Input: part model. Units: mm. Frame: model coordinates. A direction names the side the tool comes from. Coordinates: 2 decimals unless noted, no trailing zeros. Write each loop counter-clockwise with the first axis right and the second up, starting at its lowest first coordinate (ties: lowest second). Pieces come first, ordered by that corner, then holes. Notation, with made-up numbers: (51, -3.75) -> (106, -3.75) arc R19 cw to (106, 12.25) -> close; hole circle Ø11 at (28, 42.5). An arc over 180 degrees is marked (long way). Use one line per item in the form item = value. Start each with the question number.
(1) Set-up query: faces 1 (the face through (71.451, 4.504, -16.574)), 2 (the face through (-71.451, 4.504, 16.574)), 3 (the face through (1, 5, 7.5)), 4 (the face through (-1, 10, -11)). Return all of +Z, -Z, +X, -X, +Y, -Y with unobstructed straight access to the full face (end or side cutting, diameter ignored); none if empty.
(2) Cut plane A-A on z = 0. Return the cut outline in (x, y).
(3) Cut plane B-B on x = 31. Return the cut outline in (y, z), plus the area to 3 significant figures.
(4) First-contact query: pin 1 (3 mm diameter, centred on y = 5, z = 15, fed in from +X); pin 2 (3 mm diameter, centred on y = 5, z = 15, fed in from -X). Flat tips, straight axial feed; report the tip coordinate or a pass-through.
(5) Ray query, line 1 along Z through (x, y) = (71.5, 5); line 2 along Y through (x, z) = (-72.75, -15); line 3 along Z through (x, y) = (-36, 5). Return the intervals inside material, ascending.
(6) Pull-direction query (Z, two-part tool) for faces 5 (the face through (-75, 5, 0)), 6 (the face through (-67.2, 5.1, -15.3)), 7 (the face through (-1, 5, -7.5)), 8 (the face through (-1, 5, -25)); classes: released by +Z, released by -Z, zero draft, split by the parting line, or undercut.
```python
from build123d import *

# Parameters (mm, degrees)
SKETCH_1_W                       = 150
SKETCH_1_H                       = 50
EXTRUDE_1_DEPTH                  = 10
CUT_EXTRUDE_1_DEPTH              = 10
HOLE_WIZARD_M4_1_D               = 3.3
HOLE_WIZARD_M4_1_DEPTH           = 7
HOLE_WIZARD_M4_1_TIP             = 0.991420021
HOLE_WIZARD_M4_2_D               = 3.3
HOLE_WIZARD_M4_2_DEPTH           = 7
HOLE_WIZARD_M4_2_TIP             = 0.991420021
HOLE_WIZARD_M4_2_ON_FACE_2_D     = 3.3
HOLE_WIZARD_M4_2_ON_FACE_2_DEPTH = 7
HOLE_WIZARD_M4_2_ON_FACE_2_TIP   = 0.991420021


with BuildPart() as part:
    # 草图1 → 凸台-拉伸1 (new body)
    with BuildSketch(Plane(origin=(0, 0, 0), x_dir=(1, 0, 0), z_dir=(0, 1, 0))):
        Rectangle(SKETCH_1_W, SKETCH_1_H)
    extrude(amount=EXTRUDE_1_DEPTH)

    # 草图2 → 切除-拉伸1 (cut)
    with BuildSketch(Plane(origin=(0, 10, 0), x_dir=(1, 0, 0), z_dir=(0, 1, 0))):
        with BuildLine():
            Line((-55, 7.5), (55, 7.5))
            ThreePointArc((55, 7.5), (62.5, 0), (55, -7.5))
            Line((55, -7.5), (-55, -7.5))
            ThreePointArc((-55, -7.5), (-62.5, 0), (-55, 7.5))
        make_face()
    extrude(amount=-CUT_EXTRUDE_1_DEPTH, mode=Mode.SUBTRACT)

    # M4 螺纹孔的螺纹孔钻头1
    with Locations(Plane(origin=(-75, 5, -15), x_dir=(0, 0, -1), z_dir=(-1, 0, 0))):
        with Locations((0, 0), (-30, 0)):
            Hole(HOLE_WIZARD_M4_1_D / 2, depth=HOLE_WIZARD_M4_1_DEPTH)
            with Locations((0, 0, -(HOLE_WIZARD_M4_1_DEPTH + HOLE_WIZARD_M4_1_TIP / 2))):  # 118° drill point
                Cone(0, HOLE_WIZARD_M4_1_D / 2, HOLE_WIZARD_M4_1_TIP, mode=Mode.SUBTRACT)

    # M4 螺纹孔的螺纹孔钻头2
    with Locations(Plane(origin=(75, 5, 15), x_dir=(0, 0, 1), z_dir=(1, 0, 0))):
        with Locations((0, 0), (-30, 0)):
            Hole(HOLE_WIZARD_M4_2_D / 2, depth=HOLE_WIZARD_M4_2_DEPTH)
            with Locations((0, 0, -(HOLE_WIZARD_M4_2_DEPTH + HOLE_WIZARD_M4_2_TIP / 2))):  # 118° drill point
                Cone(0, HOLE_WIZARD_M4_2_D / 2, HOLE_WIZARD_M4_2_TIP, mode=Mode.SUBTRACT)

    # M4 螺纹孔的螺纹孔钻头2 on face 2
    with Locations(Plane(origin=(0, 37.698562119, 89.96356162), x_dir=(0, 0, 1), z_dir=(1, 0, 0))):
        with Locations((0, 0)):
            Hole(HOLE_WIZARD_M4_2_ON_FACE_2_D / 2, depth=HOLE_WIZARD_M4_2_ON_FACE_2_DEPTH)
            with Locations((0, 0, -(HOLE_WIZARD_M4_2_ON_FACE_2_DEPTH + HOLE_WIZARD_M4_2_ON_FACE_2_TIP / 2))):  # 118° drill point
                Cone(0, HOLE_WIZARD_M4_2_ON_FACE_2_D / 2, HOLE_WIZARD_M4_2_ON_FACE_2_TIP, mode=Mode.SUBTRACT)


solid = part.part
```
Values:
q1.face_1 = +X
q1.face_2 = -X
q1.face_3 = +Y, -Y
q1.face_4 = +Z, -Z, +X, -X, +Y
q2.outline = (-75, 0) -> (-62.5, 0) -> (-62.5, 10) -> (-75, 10) -> close; (62.5, 0) -> (75, 0) -> (75, 10) -> (62.5, 10) -> close
q3.outline = (0, -25) -> (10, -25) -> (10, -7.5) -> (0, -7.5) -> close; (0, 7.5) -> (10, 7.5) -> (10, 25) -> (0, 25) -> close
q3.area = 350 mm2
q4.pin_1 = 67.91
q4.pin_2 = -67.91
q5.line_1 = -25 to -16.65, -13.35 to 13.35, 16.65 to 25
q5.line_2 = 0 to 3.35, 6.65 to 10
q5.line_3 = -25 to -7.5, 7.5 to 25
q6.face_5 = zero draft
q6.face_6 = undercut
q6.face_7 = undercut
q6.face_8 = released by -Z
